Build history of the part. All positions in model axes, mm. A direction names the side the tool comes from. Give positions to 0.01 mm unless a question says otherwise; leave off trailing zeros. Loops run counter-clockwise (first coordinate to the right, second up) from the corner with the lowest first, then second, coordinate; pieces in that order, holes last.
1) Band-saw the part on A-A on z = 0. List the corners of the cut face in (x, y), then the cut area to 3 significant figures.
2) Band-saw the part on B-B on y = 27.6. State how many separate pieces and enclosed holes the cut face has, then the cut area to 3 significant figures.
3) Two-plate mould, pull along X, no slides. Class faces 1 (the flat face through (0, 29, 24)), 2 (the flat face through (-26.707, 28.521, -13.393)), 3 (the flat face through (-34.565, 28.521, -12.07)): +X half, -X half, draft (parallel to the pull), parting line (faces both ways), or undercut.
4) 3-axis set-ups, long thin cutter, end or side, ignore diameter. For faces 4 (the flat face through (0, 29, -22)), 5 (the flat face through (20.536, 28.521, 17.83)): which of +Z, -Z, +X, -X, +Y, -Y reach the whole face in a straight line?
5) Band-saw the part on D-D on z = 20. List the corners of the cut face in (x, y), then the cut area to 3 significant figures.
6) Band-saw the part on C-C on x = 36. List the corners of the cut face in (y, z).
7) Flat gauge pin, fed straight in: P1, Ø3, axis at x = -36, z = 0, coming from the +Y side. Where does the tip first touch, or does it go through?
8) Wall check: line 1 (Z direction, x = -10, y = 27.45); line 2 (Z direction, x = -12, y = 28); line 3 (X direction, y = 29.45, z = 10.5). Give the ranges that are in metal, low to high.
```python
from build123d import *

# Parameters (mm, degrees)
SKETCH157_R  = 1.8
PAD122_DEPTH = 3


with BuildPart() as pad122:
    # Sketch157 → Pad122 (new body)
    with BuildSketch(Plane.XZ.offset(-30)):
        with BuildLine():
            Line((-29.490381, 15), (-39.5, 9.220944))
            Line((-39.5, 9.220944), (-39.5, -9.220944))
            Line((-39.5, -9.220944), (-29.490381, -15))
            Line((-24, -11.830127), (-29.490381, -15))
            Line((-24, -11.830127), (-18.128421, -22))
            Line((-18.128421, -22), (0, -22))
            Line((0, -13.3), (0, -22))
            ThreePointArc((0, -9.7), (-1.8, -11.5), (0, -13.3))
            Line((0, -6.5), (0, -9.7))
            ThreePointArc((0, 6.5), (-6.5, 0), (0, -6.5))
            Line((0, 9.7), (0, 6.5))
            ThreePointArc((0, 13.3), (-1.8, 11.5), (0, 9.7))
            Line((0, 13.3), (0, 24))
            Line((-16.973721, 24), (0, 24))
            Line((-24, 11.830127), (-16.973721, 24))
            Line((-29.490381, 15), (-24, 11.830127))
        make_face()
        with Locations((-29, 10)):
            Circle(SKETCH157_R, mode=Mode.SUBTRACT)
        with Locations((-29, -10)):
            Circle(SKETCH157_R, mode=Mode.SUBTRACT)
        with Locations((-12, 20)):
            Circle(SKETCH157_R, mode=Mode.SUBTRACT)
        with Locations((-9.959292, 5.75)):
            Circle(SKETCH157_R, mode=Mode.SUBTRACT)
        with Locations((-9.959292, -5.75)):
            Circle(SKETCH157_R, mode=Mode.SUBTRACT)
        with Locations((-36, 0)):
            Circle(SKETCH157_R, mode=Mode.SUBTRACT)
    extrude(amount=PAD122_DEPTH)


with BuildPart() as motorcageface:
    # Part__Mirroring008: instance of Pad122
    add(pad122.part.mirror(Plane(origin=(0, 0, 0), x_dir=(0, -1, 0), z_dir=(1, 0, 0))))

    # Fusion004020015: union Pad122
    add(pad122.part)


solid = motorcageface.part
```
Findings below:
1. outline: (-39.5, 27) - (-37.8, 27) - (-37.8, 30) - (-39.5, 30) - close; (-34.2, 27) - (-6.5, 27) - (-6.5, 30) - (-34.2, 30) - close; (6.5, 27) - (34.2, 27) - (34.2, 30) - (6.5, 30) - close; (37.8, 27) - (39.5, 27) - (39.5, 30) - (37.8, 30) - close
1. area: 176 mm2
2. separate pieces: 1
2. enclosed holes: 15
2. area: 2,570 mm2
3. face 1: draft
3. face 2: undercut
3. face 3: -X half
4. face 4: -Z, +X, -X, +Y, -Y
4. face 5: +Z, +Y, -Y
5. outline: (-19.28, 27) - (-13.8, 27) - (-13.8, 30) - (-19.28, 30) - close; (-10.2, 27) - (10.2, 27) - (10.2, 30) - (-10.2, 30) - close; (13.8, 27) - (19.28, 27) - (19.28, 30) - (13.8, 30) - close
5. area: 94.1 mm2
6. outline: (27, -11.24) - (30, -11.24) - (30, -1.8) - (27, -1.8) - close; (27, 1.8) - (30, 1.8) - (30, 11.24) - (27, 11.24) - close
7. P1: passes through
8. line 1: z = -22 to -7.55, -3.95 to 3.95, 7.55 to 24
8. line 2: z = -22 to 18.2, 21.8 to 24
8. line 3: x = -37.28 to -30.73, -27.27 to -1.5, 1.5 to 27.27, 30.73 to 37.28
